Could you check a few things on this model? Use its own coordinates, in mm. A direction names the side the tool comes from. Round coordinates to 2 decimals unless told otherwise and drop trailing zeros. Write each loop counter-clockwise with the first axis right and the second up, starting at its lowest first coordinate (ties: lowest second). Pieces come first, ordered by that corner, then holes. Notation, with made-up numbers: (-38, 53) -> (-34, 53) arc R13 cw to (-34, 60) -> close; hole circle Ø1 at (85, -14.5). An arc over 180 degrees is marked (long way). Return JSON: item names as keys, results as strings.
from build123d import *

# Parameters (mm, degrees)
F0_W     = 54.107094341
F0_H     = 88.9
F1_DEPTH = 6.35
F2_W     = 54.107094341
F2_H     = 6.35
F3_DEPTH = 76.2
F4_W     = 54.107094341
F4_H     = 88.9
F5_DEPTH = 6.35
F6_R     = 4.699
F7_DEPTH = 109.22
F8_W     = 38.1
F8_H     = 6.35
F9_DEPTH = 38.1
F10_R    = 5.08


with BuildPart() as f1:
    # F0 (on Front) → F1 (new body)
    with BuildSketch(Plane.XZ):
        Rectangle(F0_W, F0_H)
    extrude(amount=F1_DEPTH)

    # F2 (on face) → F3 (join)
    with BuildSketch(Plane(origin=(0, 0, 0), x_dir=(-1, 0, 0), z_dir=(0, 1, 0))):
        with Locations((0, 41.275)):
            Rectangle(F2_W, F2_H)
    extrude(amount=F3_DEPTH)

    # F4 (on face) → F5 (join)
    with BuildSketch(Plane(origin=(0, 76.2, 0), x_dir=(-1, 0, 0), z_dir=(0, 1, 0))):
        Rectangle(F4_W, F4_H)
    extrude(amount=F5_DEPTH)

    # F6 (on face) → F7 (cut)
    with BuildSketch(Plane(origin=(0, 82.55, 0), x_dir=(-1, 0, 0), z_dir=(0, 1, 0))):
        with Locations((0, -31.75)):
            Circle(F6_R)
    extrude(amount=-F7_DEPTH, mode=Mode.SUBTRACT)

    # F8 (on face) → F9 (join)
    with BuildSketch(Plane(origin=(-27.0535471705, 0, 0), x_dir=(0, -1, 0), z_dir=(-1, 0, 0))):
        with Locations((-38.1, 41.275)):
            Rectangle(F8_W, F8_H)
    extrude(amount=F9_DEPTH)

    # F10
    f10_edges = [f1.edges().sort_by_distance(p)[0] for p in [
        (27.053547, 82.55, 0),
        (27.053547, 38.1, 44.45),
        (-27.053547, 82.55, 0),
        (-27.053547, -6.35, 0),
        (27.053547, -6.35, 0),
        (0, -6.35, -44.45),
        (0, 82.55, -44.45),
        (0, -6.35, 44.45),
        (0, 82.55, 44.45),
        (-27.053547, 69.85, 44.45),
        (-27.053547, 6.35, 44.45),
        (-65.153547, 38.1, 44.45),
        (-46.103547, 19.05, 44.45),
        (-46.103547, 57.15, 44.45),
    ]]
    fillet(f10_edges, radius=F10_R)


solid = f1.part
1) For faces 4 (the face through (0, 76.2, -3)), 5 (the face through (0, -6.35, 1)), 6 (the face through (-43.866, 55.622, 43.001)), 7 (the face through (-43.866, 20.578, 43.001)), which set-ups out of +Z, -Z, +X, -X, +Y, -Y let a thin tool reach every point of the face, with its end or its side?
Return value:
{"face 4": "-Z, +X, -X", "face 5": "+Z, -Z, +X, -X, -Y", "face 6": "+Z, -X, +Y", "face 7": "+Z, -X, -Y"}
2) I want a section at A-A, the plane z = -31.75. Please give me the cut outline in (x, y).
Return value:
{"outline": "(-27.05, -1.27) arc R5.08 ccw to (-21.97, -6.35) -> (-4.7, -6.35) -> (-4.7, 0) -> (-27.05, 0) -> close; (-27.05, 76.2) -> (-4.7, 76.2) -> (-4.7, 82.55) -> (-21.97, 82.55) arc R5.08 ccw to (-27.05, 77.47) -> close; (4.7, -6.35) -> (21.97, -6.35) arc R5.08 ccw to (27.05, -1.27) -> (27.05, 0) -> (4.7, 0) -> close; (4.7, 76.2) -> (27.05, 76.2) -> (27.05, 77.47) arc R5.08 ccw to (21.97, 82.55) -> (4.7, 82.55) -> close"}
3) I want a section at B-B, the plane x = 0. Please give me the cut outline in (y, z), and give its area (3 significant figures).
Return value:
{"outline": "(-6.35, -39.37) arc R5.08 ccw to (-1.27, -44.45) -> (0, -44.45) -> (0, -36.45) -> (-6.35, -36.45) -> close; (-6.35, -27.05) -> (0, -27.05) -> (0, 38.1) -> (76.2, 38.1) -> (76.2, -27.05) -> (82.55, -27.05) -> (82.55, 39.37) arc R5.08 ccw to (77.47, 44.45) -> (-1.27, 44.45) arc R5.08 ccw to (-6.35, 39.37) -> close; (76.2, -44.45) -> (77.47, -44.45) arc R5.08 ccw to (82.55, -39.37) -> (82.55, -36.45) -> (76.2, -36.45) -> close", "area": "1,470 mm²"}
4) If I drill on probe 1 along Y at (x, z) = (-6, 35); probe 2 along Z at (x, y) = (9.5, 7); probe 3 along X at (y, z) = (78, 3), over which ranges is the centre line in solid material (lowest first)? Write a range as [from, to].
Return value:
{"probe 1": "[-6.35, 0], [76.2, 82.55]", "probe 2": "[38.1, 44.45]", "probe 3": "[-27.03, 27.03]"}
5) Will these pins go through, and if not, where does the flat tip stop? pin 1 Ø6 at (x, y) = (13, 59.5) entering from -Z; pin 2 Ø0.6 at (x, z) = (-52, 38.5) entering from -Y; pin 3 Ø22.5 at (y, z) = (6, -15.5) entering from -X.
Return value:
{"pin 1": "z = 38.1", "pin 2": "y = 19.05", "pin 3": "x = -27.05"}
6) I want a section at D-D, the plane x = -31. Please give me the cut outline in (y, z), and give its area (3 significant figures).
Return value:
{"outline": "(19.05, 38.1) -> (57.15, 38.1) -> (57.15, 39.37) arc R5.08 ccw to (52.07, 44.45) -> (24.13, 44.45) arc R5.08 ccw to (19.05, 39.37) -> close", "area": "231 mm²"}
7) I want a section at C-C, the plane y = 12. Please give me the cut outline in (x, z).
Return value:
{"outline": "(-27.05, 38.1) -> (27.05, 38.1) -> (27.05, 39.37) arc R5.08 ccw to (21.97, 44.45) -> (-21.97, 44.45) arc R5.08 ccw to (-27.05, 39.37) -> close"}
8) Thinking about a two-plate mould opening in X: for faces 1 (the face through (0.61, 79.42, -27.09)), 2 (the face through (-8, 38, 38.1)), 3 (the face through (-25.53, -4.9, -1.95)), which applies, pulls with the +X half, pulls with the -X half, needs draft (parallel to the pull), parting line crosses it, or undercut?
Return value:
{"face 1": "undercut", "face 2": "needs draft", "face 3": "pulls with the -X half"}
